For this review, take the finished solid that the model builds, in its own axes (mm). Face numbers are marked on the shaded views. A direction names the side the tool comes from. Give positions to 0.01 mm unless a question says otherwise; leave off trailing zeros. Loops run counter-clockwise (first coordinate to the right, second up) from the corner with the lowest first, then second, coordinate; pieces in that order, holes last. Notation, with made-up numbers: (-27.5, 62) - (27.5, 62) arc R29 ccw to (27.5, 91) - close; hole circle Ø5 at (13.25, 82.5). An arc over 180 degrees is marked (long way). Answer in a Markdown table with one row per item.
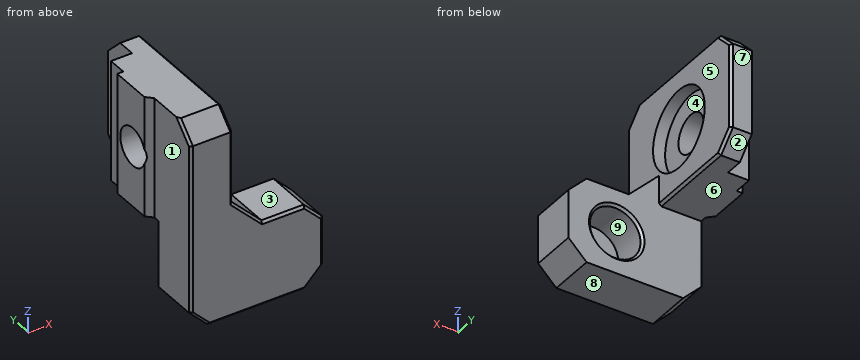
```python
from build123d import *

# Parameters (mm, degrees)
CYLINDER_R        = 4.2
CYLINDER_DEPTH    = 10
CYLINDER001_R     = 6.5
CYLINDER001_DEPTH = 10
CYLINDER002_R     = 3.15
CYLINDER002_DEPTH = 10
BOX002_W          = 3.5
BOX002_H          = 8
BOX002_DEPTH      = 20
BOX001_W          = 7
BOX001_H          = 26
BOX001_DEPTH      = 20
CHAMFER004_SIZE   = 3
BOX003_W          = 2
BOX003_H          = 7.8
BOX003_DEPTH      = 20
CHAMFER003_SIZE   = 1
BOX_W             = 22
BOX_H             = 8
BOX_DEPTH         = 14
CHAMFER_SIZE      = 3
CHAMFER005_SIZE   = 5
CHAMFER006_SIZE   = 0.4


with BuildPart() as cylinder:
    # Cylinder → Cylinder (new body)
    with BuildSketch(Plane(origin=(14, 4, 7), x_dir=(1, 0, 0), z_dir=(0, 1, 0))):
        Circle(CYLINDER_R)
    extrude(amount=CYLINDER_DEPTH)


with BuildPart() as cylinder001:
    # Cylinder001 → Cylinder001 (new body)
    with BuildSketch(Plane(origin=(5, 15, 24), x_dir=(0, 0, -1), z_dir=(1, 0, 0))):
        Circle(CYLINDER001_R)
    extrude(amount=CYLINDER001_DEPTH)


with BuildPart() as fusion001:
    # Cylinder002 → Cylinder002 (new body)
    with BuildSketch(Plane(origin=(-2, 15, 24), x_dir=(0, 0, -1), z_dir=(1, 0, 0))):
        Circle(CYLINDER002_R)
    extrude(amount=CYLINDER002_DEPTH)

    # Fusion001: union Cylinder001
    add(cylinder001.part)


with BuildPart() as cube002:
    # Box002 → Box002 (new body)
    with BuildSketch(Plane(origin=(0, 22, 14), x_dir=(1, 0, 0), z_dir=(0, 0, 1))):
        with Locations((1.75, 4)):
            Rectangle(BOX002_W, BOX002_H)
    extrude(amount=BOX002_DEPTH)


with BuildPart() as chamfer004:
    # Box001 → Box001 (new body)
    with BuildSketch(Plane(origin=(0, 2, 14), x_dir=(1, 0, 0), z_dir=(0, 0, 1))):
        with Locations((3.5, 13)):
            Rectangle(BOX001_W, BOX001_H)
    extrude(amount=BOX001_DEPTH)

    # Cut: cut Cube002
    add(cube002.part, mode=Mode.SUBTRACT)

    # Chamfer004
    chamfer004_edges = [chamfer004.edges().sort_by_distance(p)[0] for p in [
        (5.25, 28, 34),
        (3.5, 2, 34),
        (5.25, 28, 14),
    ]]
    chamfer(chamfer004_edges, length=CHAMFER004_SIZE)


with BuildPart() as chamfer003:
    # Box003 → Box003 (new body)
    with BuildSketch(Plane(origin=(-1, 11.1, 14), x_dir=(1, 0, 0), z_dir=(0, 0, 1))):
        with Locations((1, 3.9)):
            Rectangle(BOX003_W, BOX003_H)
    extrude(amount=BOX003_DEPTH)

    # Chamfer003
    chamfer003_edges = [chamfer003.edges().sort_by_distance(p)[0] for p in [
        (-1, 11.1, 24),
    ]]
    chamfer(chamfer003_edges, length=CHAMFER003_SIZE)


with BuildPart() as chamfer006:
    # Box → Box (new body)
    with BuildSketch(Plane(origin=(0, 2, 0), x_dir=(1, 0, 0), z_dir=(0, 0, 1))):
        with Locations((11, 4)):
            Rectangle(BOX_W, BOX_H)
    extrude(amount=BOX_DEPTH)

    # Chamfer
    chamfer_edges = [chamfer006.edges().sort_by_distance(p)[0] for p in [
        (0, 6, 0),
        (22, 6, 14),
        (22, 6, 0),
    ]]
    chamfer(chamfer_edges, length=CHAMFER_SIZE)

    # Fusion: union Chamfer004, Chamfer003
    add(chamfer004.part)
    add(chamfer003.part)

    # Chamfer005
    chamfer005_edges = [chamfer006.edges().sort_by_distance(p)[0] for p in [
        (7, 6, 14),
    ]]
    chamfer(chamfer005_edges, length=CHAMFER005_SIZE)

    # Cut010011008009003016026008002: cut Fusion001
    add(fusion001.part, mode=Mode.SUBTRACT)

    # Cut010011008009003016026008003: cut Cylinder
    add(cylinder.part, mode=Mode.SUBTRACT)

    # Chamfer006
    chamfer006_edges = [chamfer006.edges().sort_by_distance(p)[0] for p in [
        (15.5, 2, 14),
        (20.5, 2, 12.5),
        (22, 2, 7),
        (20.5, 2, 1.5),
        (11, 2, 0),
        (1.5, 2, 1.5),
        (9.8, 10, 7),
        (9.5, 2, 16.5),
        (7, 2, 25),
        (7, 3.5, 32.5),
        (7, 15, 34),
        (7, 17.5, 14),
        (7, 26.5, 32.5),
        (7, 26.5, 15.5),
        (7, 28, 24),
        (0, 3.5, 32.5),
        (0, 2, 17),
    ]]
    chamfer(chamfer006_edges, length=CHAMFER006_SIZE)


solid = chamfer006.part
```
1. We need section A-A, the plane y = 15. Give the boundary of the cut face in (x, z).
Values:
| item | result |
|---|---|
| outline | (-1, 14) - (6.6, 14) - (7, 14.4) - (7, 17.5) - (5, 17.5) - (5, 20.85) - (-1, 20.85) - close; (-1, 27.15) - (5, 27.15) - (5, 30.5) - (7, 30.5) - (7, 33.6) - (6.6, 34) - (-1, 34) - close |
2. Mouldability with a two-part tool opening along Z and no side actions: class the marked faces 1, 2, 3 and 4 as released by +Z, released by -Z, zero draft, split by the parting line, or undercut.
Values:
| item | result |
|---|---|
| face 1 | zero draft |
| face 2 | released by -Z |
| face 3 | released by +Z |
| face 4 | undercut |
3. We need section D-D, the plane x = 14. Give the boundary of the cut face in (y, z).
Values:
| item | result |
|---|---|
| outline | (2, 0.4) - (2.4, 0) - (10, 0) - (10, 2.4) - (9.6, 2.8) - (4, 2.8) - (4, 11.2) - (9.6, 11.2) - (10, 11.6) - (10, 14) - (2.4, 14) - (2, 13.6) - close |
4. Wall thickness on line 1 (X direction, y = 8.5, z = 7); line 2 (Z direction, x = 5.6, y = 15); line 3 (Y direction, x = 1.5, z = 24): over which ranges is each line inside the solid? List them lowest first. Write a range as [from, to].
Values:
| item | result |
|---|---|
| line 1 | x = [0, 9.8], [18.2, 22] |
| line 2 | z = [14, 17.5], [30.5, 34] |
| line 3 | y = [2, 11.85], [18.15, 22] |
5. Clearance check with flat-ended pins moving along their axes: pin 1 (1 mm diameter, centred on x = 18, y = 7.5, fed in from +Z); pin 2 (3 mm diameter, centred on x = 1.5, z = 27, fed in from +Y); pin 3 (8.5 mm diameter, centred on x = 3.5, y = 14.5, fed in from -Z); pin 4 (5 mm diameter, centred on x = 2, z = 16.5, fed in from +Y). State where each tip first meets the part, or that it passes through.
Values:
| item | result |
|---|---|
| pin 1 | stops at z = 14 |
| pin 2 | stops at y = 22 |
| pin 3 | stops at z = 14 |
| pin 4 | stops at y = 28 |
6. For the marked faces 5, 6, 7, 8 and 9, list the 3-axis set-ups (+Z, -Z, +X, -X, +Y, -Y) from which the entire face can be reached by the end or side of a thin tool; tool diameter is ignored.
Values:
| item | result |
|---|---|
| face 5 | +Z, +X, +Y |
| face 6 | -Z, +X, -X, +Y |
| face 7 | +Z, -Z, +X, -X, +Y |
| face 8 | -Z, +X, -X, +Y, -Y |
| face 9 | +Y |
7. We need section C-C, the plane z = 7. Give the boundary of the cut face in (x, y), and give its area (3 significant figures).
Values:
| item | result |
|---|---|
| outline | (0, 2.4) - (0.4, 2) - (21.6, 2) - (22, 2.4) - (22, 10) - (18.6, 10) - (18.2, 9.6) - (18.2, 4) - (9.8, 4) - (9.8, 9.6) - (9.4, 10) - (0, 10) - close |
| area | 125 mm^2 |
8. We need section B-B, the plane z = 24. Give the boundary of the cut face in (x, y), and give its area (3 significant figures).
Values:
| item | result |
|---|---|
| outline | (-1, 18.15) - (5, 18.15) - (5, 21.5) - (7, 21.5) - (7, 27.6) - (6.6, 28) - (3.5, 28) - (3.5, 22) - (0, 22) - (0, 18.9) - (-1, 18.9) - close; (-0.75, 11.85) - (0, 11.1) - (0, 2.4) - (0.4, 2) - (6.6, 2) - (7, 2.4) - (7, 8.5) - (5, 8.5) - (5, 11.85) - close |
| area | 104 mm^2 |
